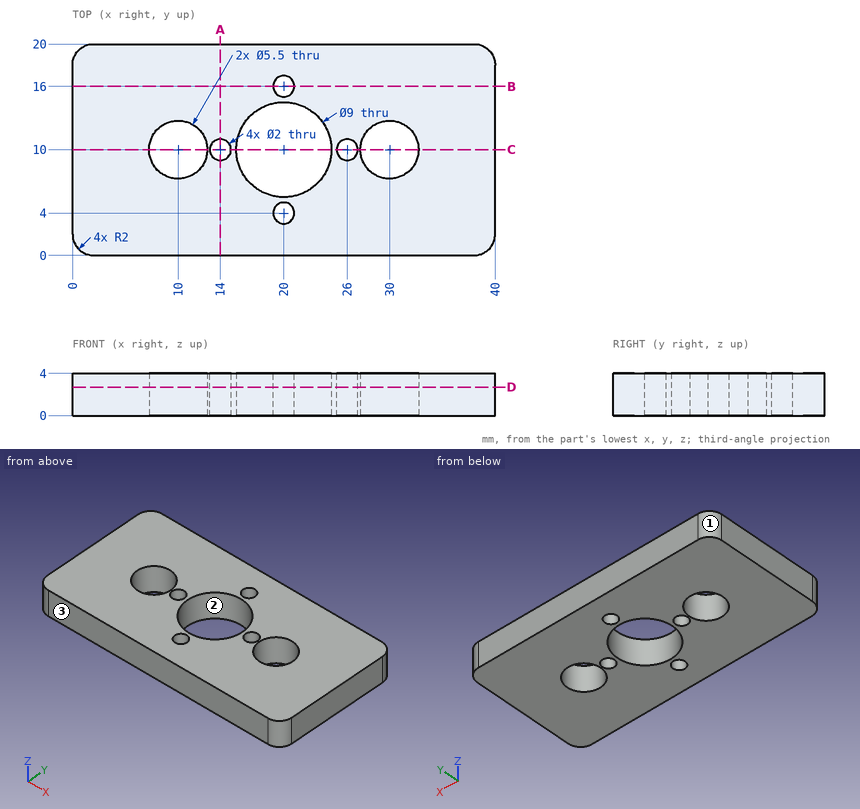
Geometry check sheet. Reference: drawing and pictorial views, mm from the part's lowest x, y, z. Coordinates: 2 decimals unless noted, no trailing zeros. Write each loop counter-clockwise with the first axis right and the second up, starting at its lowest first coordinate (ties: lowest second). Pieces come first, ordered by that corner, then holes. Notation, with made-up numbers: (-8.75, 18.25) -> (5.25, 18.25) arc R20 cw to (5.25, 34.25) -> close; hole circle Ø5 at (11.25, 60). An arc over 180 degrees is marked (long way). One line per question, with ' | ' between items.
1. Cross-section at A-A on x = 14. Record the cut outline in (y, z), and give its area (3 significant figures).
Answers:
outline: (0, 0) -> (9, 0) -> (9, 4) -> (0, 4) -> close; (11, 0) -> (20, 0) -> (20, 4) -> (11, 4) -> close | area: 72.0 mm²
2. Depth check by flat-ended pin: pin 1 Ø1.5 at (x, z) = (13.5, 2) entering from -Y; pin 2 Ø1.6 at (x, y) = (14, 10) entering from -Z. Enter the tip coordinate at first touch or a pass-through.
Answers:
pin 1: stops at y = 0 | pin 2: passes through
3. Thickness scan on probe 1 along Y at (x, z) = (20, 1.9); probe 2 along Y at (x, z) = (8, 3); probe 3 along Y at (x, z) = (10, 1.35). Record the ranges inside material, lowest first. Write a range as from..to.
Answers:
probe 1: y = 0..3, 5..5.5, 14.5..15, 17..20 | probe 2: y = 0..8.11, 11.89..20 | probe 3: y = 0..7.25, 12.75..20
4. Cross-section at D-D on z = 2.7. Record the cut outline in (x, y), and give its area (3 significant figures).
Answers:
outline: (0, 2) arc R2 ccw to (2, 0) -> (38, 0) arc R2 ccw to (40, 2) -> (40, 18) arc R2 ccw to (38, 20) -> (2, 20) arc R2 ccw to (0, 18) -> close; hole circle Ø5.5 at (10, 10); hole circle Ø2 at (14, 10); hole circle Ø9 at (20, 10); hole circle Ø2 at (20, 4); hole circle Ø2 at (20, 16); hole circle Ø2 at (26, 10); hole circle Ø5.5 at (30, 10) | area: 673 mm²
5. Cross-section at B-B on y = 16. Record the cut outline in (x, z), and give its area (3 significant figures).
Answers:
outline: (0, 0) -> (19, 0) -> (19, 4) -> (0, 4) -> close; (21, 0) -> (40, 0) -> (40, 4) -> (21, 4) -> close | area: 152 mm²
6. Draft check along X on the marked faces 1, 2 and 3. Enter one of: +X half, -X half, draft (parallel to the pull), parting line (faces both ways), or undercut.
Answers:
face 1: -X half | face 2: undercut | face 3: draft
7. Cross-section at C-C on y = 10. Record the cut outline in (x, z).
Answers:
outline: (0, 0) -> (7.25, 0) -> (7.25, 4) -> (0, 4) -> close; (12.75, 0) -> (13, 0) -> (13, 4) -> (12.75, 4) -> close; (15, 0) -> (15.5, 0) -> (15.5, 4) -> (15, 4) -> close; (24.5, 0) -> (25, 0) -> (25, 4) -> (24.5, 4) -> close; (27, 0) -> (27.25, 0) -> (27.25, 4) -> (27, 4) -> close; (32.75, 0) -> (40, 0) -> (40, 4) -> (32.75, 4) -> close
